Autodesk Inventor part; units mm, degrees
ref_plane "YZ Plane" through (0, 0, 0) normal (1, 0, 0) x (0, 1, 0)
ref_plane "XZ Plane" through (0, 0, 0) normal (0, 1, 0) x (-1, 0, 0)
ref_plane "XY Plane" through (0, 0, 0) normal (0, 0, 1) x (1, 0, 0)
sketch "Sketch1" plane through (0, 0, 0) normal (0, 0, 1) x (1, 0, 0)
  line L0 (-11.0744, 5.588) -> (11.0744, 5.588)
  line L1 (11.0744, 5.588) -> (11.0744, -5.588)
  line L2 (11.0744, -5.588) -> (-11.0744, -5.588)
  line L3 (-11.0744, -5.588) -> (-11.0744, 5.588)
  circle A0 centre (-8.3312, 2.4384) radius 1.3462
  circle A1 centre (8.3312, 2.4384) radius 1.3462
  circle A2 centre (8.3312, -2.794) radius 1.3462
  circle A3 centre (-8.3312, -2.794) radius 1.3462
  line L4 (0, -3.2143) -> (0, 3.2143) construction
  line L5 (1.4766, -3.2143) -> (1.4766, 3.2143)
  line L6 (-1.4766, 3.2143) -> (-1.4766, -3.2143)
  arc A4 (-1.4766, -3.2143) -> (1.4766, -3.2143) centre (0, -3.2143) ccw
  arc A5 (1.4766, 3.2143) -> (-1.4766, 3.2143) centre (0, 3.2143) ccw
  point P0 (0, 0)
  dimension "d0" = 22.1488
  dimension "d1" = 11.176
  dimension "d2" = 2.6924
  dimension "d3" = 2.6924
  dimension "d4" = 2.6924
  dimension "d5" = 2.6924
  dimension "d6" = 3.1496
  dimension "d7" = 2.794
  dimension "d8" = 5.2324
  dimension "d9" = 2.7432
  dimension "d10" = 2.7432
  dimension "d11" = 3.1496
  dimension "d12" = 2.794
extrude "Extrusion1" add sketch "Sketch1" along normal blind 1.5494 contours L0 L1 L2 L3 | A4 L6 A5 L5
sketch "Sketch2" plane through (-11.0744, -5.588, 0) normal (0, -1, 0) x (1, 0, 0)
  line L0 (5.5567, 1.5494) -> (16.6565, 1.5494)
  line L1 (16.6565, 1.5494) -> (16.6565, 0)
  line L2 (16.6565, 0) -> (5.5567, 0)
  line L3 (5.5567, 0) -> (5.5567, 1.5494)
  line L4 (22.1488, 0) -> (22.1488, 1.5494)
  line L5 (0, 0) -> (0, 1.5494)
  line L6 (22.1488, 1.5494) -> (0, 1.5494)
  line L7 (0, 0) -> (22.1488, 0)
  point P0 (11.0744, 0)
  dimension "d15" = 11.0998
  dimension "d16" = 1.5494
extrude "Extrusion2" add sketch "Sketch2" along normal blind 3.3782 contours L0 L1 L2 L3
sketch "Sketch3" plane through (-5.5177, -5.588, 1.5494) normal (0, 0, 1) x (1, 0, 0)
  line L0 (0, -3.3559) -> (11.0998, -3.3559)
  line L1 (11.0998, -3.3559) -> (11.0998, -4.8799)
  line L2 (11.0998, -4.8799) -> (0, -4.8799)
  line L3 (0, -4.8799) -> (0, -3.3559)
  point P0 (5.5177, 5.588)
  dimension "d19" = 11.0998
  dimension "d20" = 1.524
extrude "Extrusion3" add sketch "Sketch3" along normal blind 6.4008
sketch "Sketch4" plane through (-5.5177, -8.9439, 1.5494) normal (0, 1, 0) x (1, 0, 0)
  line L0 (13.7962, -29.1915) -> (-3.1964, -29.1915)
  line L1 (-3.1964, -6.3061) -> (13.7962, -6.3061)
  line L2 (-5.5567, 1.5494) -> (16.5921, 1.5494)
  arc A0 (-5.7364, -22.2822) -> (-5.7364, -13.2153) centre (-5.7998, -17.7488) ccw
  arc A1 (16.3362, -13.2152) -> (16.3362, -22.2823) centre (16.3912, -17.7488) ccw
  line L3 (16.3362, -8.8461) -> (16.3362, -13.2152)
  line L4 (16.3362, -22.2823) -> (16.3362, -26.6515)
  line L5 (-5.7364, -26.6515) -> (-5.7364, -22.2822)
  line L6 (-5.7364, -13.2153) -> (-5.7364, -8.8461)
  circle A2 centre (5.2999, -17.7488) radius 4.9657
  arc A3 (13.7962, -29.1915) -> (16.3362, -26.6515) centre (13.7962, -26.6515) ccw
  arc A4 (-5.7364, -26.6515) -> (-3.1964, -29.1915) centre (-3.1964, -26.6515) ccw
  arc A5 (16.3362, -8.8461) -> (13.7962, -6.3061) centre (13.7962, -8.8461) ccw
  arc A6 (-3.1964, -6.3061) -> (-5.7364, -8.8461) centre (-3.1964, -8.8461) ccw
  circle A7 centre (13.7962, -26.6515) radius 1.3208
  circle A8 centre (13.7962, -8.5679) radius 1.3208
  circle A9 centre (-3.1964, -8.5679) radius 1.3208
  circle A10 centre (-3.1964, -26.6515) radius 1.3208
  point P0 (5.5177, 1.5494)
  point P1 (-5.7364, -6.3061)
  point P2 (-5.7364, -29.1915)
  point P3 (16.3362, -6.3061)
  point P4 (5.5177, 1.5494)
  point P5 (16.3362, -17.7488)
  point P6 (5.5177, 1.5494)
  dimension "d25" = 9.0678
  dimension "d26" = 9.0678
  dimension "d27" = 9.9314
  dimension "d28" = 2.54
  dimension "d29" = 2.6416
  dimension "d30" = 2.6416
  dimension "d31" = 2.6416
  dimension "d32" = 2.6416
  dimension "d33" = 2.54
extrude "Extrusion4" add sketch "Sketch4" against normal blind 1.524
sketch "Sketch5" plane through (-11.0744, -8.9662, 0) normal (0, -1, 0) x (1, 0, 0)
  line L0 (16.6565, 1.5494) -> (5.5567, 1.5494)
  line L1 (5.5567, 1.5494) -> (5.5567, 0)
  line L2 (5.5567, 0) -> (16.6565, 0)
  line L3 (16.6565, 0) -> (16.6565, 1.5494)
  point P0 (11.0744, 0)
extrude "Extrusion5" add sketch "Sketch5" along normal blind 1.5016
fillet "Fillet1" radius 3.175 1 edges at (0.0322, -10.4678, 0)
sketch "Sketch6" plane through (0, 0, 0) normal (0, 0, -1) x (-1, 0, 0)
  line L0 (0, -3.2139) -> (0, 3.2139) construction
  line L1 (1.4732, -3.2139) -> (1.4732, 3.2139)
  line L2 (-1.4732, 3.2139) -> (-1.4732, -3.2139)
  arc A0 (-1.4732, -3.2139) -> (1.4732, -3.2139) centre (0, -3.2139) ccw
  arc A1 (1.4732, 3.2139) -> (-1.4732, 3.2139) centre (0, 3.2139) ccw
  point P0 (0, 0)
  dimension "d41" = 2.9464
extrude "Extrusion6" cut sketch "Sketch6" against normal blind 9.4615
equation "\"BendRadius\" = Thickness"
equation "\"BendReliefWidth\" = Thickness"
equation "\"BendReliefDepth\" = 0.5 * Thickness"
equation "\"CornerReliefSize\" = 4 * Thickness"
equation "\"MinimumRemnant\" = 2 * Thickness"
equation "\"TransitionRadius\" = BendRadius"
equation "\"JacobiRadiusSize\" = Thickness"
equation "\"GapSize\" = Thickness"
properties part number "motor mount complete"
The model under review builds one solid part; all positions refer to its coordinate system, in mm. A direction names the side the tool comes from. Round coordinates to 2 decimals unless told otherwise and drop trailing zeros. Loops run counter-clockwise (first coordinate to the right, second up) from the corner with the lowest first, then second, coordinate; pieces in that order, holes last. Notation, with made-up numbers: (-35, -22) -> (0, -22) arc R22 cw to (0, 11) -> close; hole circle Ø9 at (30, -32). An arc over 180 degrees is marked (long way). Return JSON: item names as keys, results as strings.
(1) Add section C-C on y = -2. Write out the cut boundary in (x, z).
Solved:
{"outline": "(-11.07, 0) -> (-9.42, 0) -> (-9.42, 1.55) -> (-11.07, 1.55) -> close; (-7.24, 0) -> (-1.47, 0) -> (-1.47, 1.55) -> (-7.24, 1.55) -> close; (1.47, 0) -> (7.24, 0) -> (7.24, 1.55) -> (1.47, 1.55) -> close; (9.42, 0) -> (11.07, 0) -> (11.07, 1.55) -> (9.42, 1.55) -> close"}
(2) Add section A-A on y = 0.25. Write out the cut boundary in (x, z), plus the area to 3 significant figures.
Solved:
{"outline": "(-11.07, 0) -> (-1.47, 0) -> (-1.47, 1.55) -> (-11.07, 1.55) -> close; (1.47, 0) -> (11.07, 0) -> (11.07, 1.55) -> (1.47, 1.55) -> close", "area": "29.8 mm2"}
(3) For line 1 (Z direction, x = 6.75, y = 4.25); line 2 (Y direction, x = 9.75, z = 29); line 3 (Y direction, x = -1, z = 2), list the stretches that pass through material, from the lowest coordinate up.
Solved:
{"line 1": "0 to 1.55", "line 2": "-10.47 to -8.94", "line 3": "-10.24 to -8.94"}
(4) Add section B-B on z = 16. Write out the cut boundary in (x, y), plus the area to 3 significant figures.
Solved:
{"outline": "(-8.21, -10.47) -> (-3.93, -10.47) -> (-3.93, -8.94) -> (-8.21, -8.94) -> close; (3.49, -10.47) -> (7.76, -10.47) -> (7.76, -8.94) -> (3.49, -8.94) -> close", "area": "13.0 mm2"}
(5) Add section D-D on x = 0. State how many separate pieces and enclosed holes the cut face has, plus the area to 3 significant figures.
Solved:
{"separate pieces": "3", "enclosed holes": "0", "area": "37.6 mm2"}
(6) For pin 1 (1.2 mm diameter, centred on y = 0, z = 0.5, fed in from -X); pin 2 (5.5 mm diameter, centred on y = -7.5, z = 5, fed in from -X); pin 3 (1.7 mm diameter, centred on y = -9.5, z = 13, fed in from +X), all flat-tipped, find the tip position at first contact; note any pin that passes through.
Solved:
{"pin 1": "x = -11.07", "pin 2": "x = -5.52", "pin 3": "x = 10.82"}
(7) The part is to be moulded in two halves that separate along X. For faces 6 (the flat face through (2, -2, 1.549)), 7 (the cylindrical face through (-7.088, -2.278, 0.764)), 8 (the cylindrical face through (-6.785, -9.695, 19.397)), say which applies: released by +X, released by -X, zero draft, split by the parting line, or undercut.
Solved:
{"face 6": "zero draft", "face 7": "undercut", "face 8": "released by -X"}
(8) For faces 1 (the flat face through (8, -5.588, 1)), 2 (the flat face through (-7, -10, 7.856)), 3 (the flat face through (7, -10, 7.856)), 4 (the flat face through (-8, -5.588, 1)), 5 (the flat face through (1.473, 0, 1)), list the 3-axis set-ups (+Z, -Z, +X, -X, +Y, -Y) from which the entire face can be reached by the end or side of a thin tool; tool diameter is ignored.
Solved:
{"face 1": "+Z, -Z, +X, -Y", "face 2": "-Z, -X, +Y, -Y", "face 3": "-Z, +X, +Y, -Y", "face 4": "+Z, -Z, -X, -Y", "face 5": "+Z, -Z"}
